Can you work these out from the model? Positions are in its coordinate system, mm. A direction names the side the tool comes from. Round coordinates to 2 decimals unless told otherwise and drop trailing zeros. Loops run counter-clockwise (first coordinate to the right, second up) from the corner with the lowest first, then second, coordinate; pieces in that order, holes last. Notation, with made-up numbers: (34, 34) -> (84, 34) arc R16 cw to (84, 62) -> close; hole circle Ø3 at (27, -24.75). An arc over 180 degrees is marked (long way). Answer as a JSON object with one key per item and string values.
```python
from build123d import *
from build123d.topology import SkipClean

# Parameters (mm, degrees)
SKETCH1_W           = 120
SKETCH1_H           = 20
BOSS_EXTRUDE1_DEPTH = 6
CUT_EXTRUDE1_DEPTH  = 4.6
SKETCH3_R           = 3.4
CUT_EXTRUDE2_DEPTH  = 4.6
SKETCH4_R           = 2
CUT_EXTRUDE3_DEPTH  = 122.803119829
FILLET1_R           = 0.6


with BuildPart() as part:
    # Sketch1 → Boss-Extrude1 (new body)
    with BuildSketch(Plane(origin=(0, 0, 0), x_dir=(1, 0, 0), z_dir=(0, 1, 0))):
        with Locations((60, 10)):
            Rectangle(SKETCH1_W, SKETCH1_H)
    extrude(amount=BOSS_EXTRUDE1_DEPTH)

    # Sketch2 → Cut-Extrude1 (cut)
    with BuildSketch(Plane(origin=(0, 6, 0), x_dir=(1, 0, 0), z_dir=(0, 1, 0))):
        with BuildLine():
            Line((93.674922601, 11.942124585), (109.694736842, 13.386268507))
            ThreePointArc((109.694736842, 13.386268507), (113.4, 10), (109.694736842, 6.613731493))
            Line((109.694736842, 6.613731493), (93.674922601, 8.057875415))
            ThreePointArc((93.674922601, 8.057875415), (91.9, 10), (93.674922601, 11.942124585))
        make_face()
    extrude(amount=-CUT_EXTRUDE1_DEPTH, mode=Mode.SUBTRACT)

    # Sketch3 → Cut-Extrude2 (cut)
    with SkipClean():  # the faces are left unmerged after this step: merging them gives an invalid solid
        with BuildSketch(Plane(origin=(0, 1.4, 0), x_dir=(1, 0, 0), z_dir=(0, 1, 0))):
            with Locations(Location((110, 10, 0), (0, 0, 264.848860425))):
                Circle(SKETCH3_R)
        extrude(amount=-CUT_EXTRUDE2_DEPTH, mode=Mode.SUBTRACT)

    # Sketch4 → Cut-Extrude3 (cut, through all)
    with SkipClean():  # the faces are left unmerged after this step: merging them gives an invalid solid
        with BuildSketch(Plane(origin=(0, 6, 0), x_dir=(1, 0, 0), z_dir=(0, 1, 0))):
            with Locations(Location((10, 10, 0), (0, 0, 270))):
                Circle(SKETCH4_R)
        extrude(amount=-CUT_EXTRUDE3_DEPTH, mode=Mode.SUBTRACT)

    # Fillet1
    fillet1_edges = [part.edges().sort_by_distance(p)[0] for p in [
        (120, 6, -10),
        (60, 6, -20),
        (0, 6, -10),
        (60, 0, -20),
        (120, 0, -10),
        (60, 0, 0),
        (0, 0, -10),
        (60, 6, 0),
    ]]
    fillet(fillet1_edges, radius=FILLET1_R)


solid = part.part
```
Q1. I'm going to push flat-ended pins straight in: pin 1 (4 mm diameter, centred on x = 110, z = -10, fed in from +Y); pin 2 (2 mm diameter, centred on x = 100, z = -9.5, fed in from +Y). Where does each tip first touch, or does it pass through?
Determined:
{"pin 1": "through", "pin 2": "y = 1.4"}
Q2. I want a section at C-C, the plane x = 10. Write out the boundary of the cut face in (y, z), then the cut area to 3 significant figures.
Determined:
{"outline": "(0, -19.4) arc R0.6 ccw to (0.6, -20) -> (5.4, -20) arc R0.6 ccw to (6, -19.4) -> (6, -12) -> (0, -12) -> close; (0, -8) -> (6, -8) -> (6, -0.6) arc R0.6 ccw to (5.4, 0) -> (0.6, 0) arc R0.6 ccw to (0, -0.6) -> close", "area": "95.7 mm²"}
Q3. I want a section at B-B, the plane z = -10. Write out the boundary of the cut face in (x, y).
Determined:
{"outline": "(0, 0.6) arc R0.6 ccw to (0.6, 0) -> (8, 0) -> (8, 6) -> (0.6, 6) arc R0.6 ccw to (0, 5.4) -> close; (12, 0) -> (106.6, 0) -> (106.6, 1.4) -> (91.9, 1.4) -> (91.9, 6) -> (12, 6) -> close; (113.4, 0) -> (119.4, 0) arc R0.6 ccw to (120, 0.6) -> (120, 5.4) arc R0.6 ccw to (119.4, 6) -> (113.4, 6) -> close"}
Q4. We'd pull the mould along Z, two halves only. Please class faces 3 (the flat face through (59, 3, -20)), 4 (the flat face through (101, 1.4, -10)), 5 (the flat face through (101.797, 3.732, -7.326)), 6 (the flat face through (0, 3, -10)): pulls with the +Z half, pulls with the -Z half, needs draft (parallel to the pull), parting line crosses it, or undercut.
Determined:
{"face 3": "pulls with the -Z half", "face 4": "undercut", "face 5": "undercut", "face 6": "needs draft"}
Q5. On a 3-axis mill with a long thin cutter (end or side, diameter ignored), from which of +Z, -Z, +X, -X, +Y, -Y can I reach the whole of each face in a straight line? I mean faces 1 (the flat face through (59, 3, 0)), 2 (the flat face through (101.573, 3.732, -12.654)). Say none if no direction works.
Determined:
{"face 1": "+Z, +X, -X, +Y, -Y", "face 2": "+Y"}
Q6. If I drill on L1, parallel to X at y = 1.25, z = -10; L2, parallel to X at y = 3.65, z = -10; L3, parallel to Z at x = 110, y = 0.5, over which ranges is the centre line in solid material (lowest first)? Write a range as [from, to].
Determined:
{"L1": "[0, 8], [12, 106.6], [113.4, 120]", "L2": "[0, 8], [12, 91.9], [113.4, 120]", "L3": "[-19.99, -13.4], [-6.6, -0.01]"}
Q7. I want a section at A-A, the plane y = 4.4. Write out the boundary of the cut face in (x, z), then the cut area to 3 significant figures.
Determined:
{"outline": "(0, -20) -> (120, -20) -> (120, 0) -> (0, 0) -> close; hole circle Ø4 at (10, -10); hole (93.67, -11.94) -> (109.69, -13.39) arc R3.4 ccw (long way) to (109.69, -6.61) -> (93.67, -8.06) arc R1.95 ccw to start", "area": "2,280 mm²"}
